from build123d import *

# Parameters (mm, degrees)
BOSS_EXTRUDE1_DEPTH = 2


with BuildPart() as part:
    # Sketch1 → Boss-Extrude1 (new body)
    with BuildSketch(Plane.XY):
        with BuildLine():
            Line((5, 6.009754879), (-15, 6.009754879))
            ThreePointArc((-15, 6.009754879), (-21.009754879, 0), (-15, -6.009754879))
            Line((-15, -6.009754879), (5, -6.009754879))
            Line((5, -6.009754879), (5, 6.009754879))
        make_face()
        with BuildLine():
            ThreePointArc((-12.450490243, -2.75), (-18.75, 0), (-12.450490243, 2.75))
            Line((-12.450490243, 2.75), (0, 2.25))
            ThreePointArc((0, 2.25), (1.590990258, 1.590990258), (2.25, 0))
            ThreePointArc((2.25, 0), (1.590990258, -1.590990258), (0, -2.25))
            Line((0, -2.25), (-12.450490243, -2.75))
        make_face(mode=Mode.SUBTRACT)
    extrude(amount=BOSS_EXTRUDE1_DEPTH)


solid = part.part
Check sheet for the modelled part. Datum: model origin and axes. Units: mm. A direction names the side the tool comes from. Coordinates: 2 decimals unless noted, no trailing zeros. Loops run counter-clockwise (first coordinate to the right, second up) from the corner with the lowest first, then second, coordinate; pieces in that order, holes last. Notation, with made-up numbers: (1, 86.25) -> (42, 86.25) arc R18 cw to (42, 117.25) -> close; hole circle Ø4 at (-10.5, 5). An arc over 180 degrees is marked (long way). Answer in a Markdown table with one row per item.
1. Release check for a two-part mould opening along X. For faces 3 (the face through (-6.312, 2.504, 0.986)), 4 (the face through (-5, 6.01, 1)), 5 (the face through (-21.01, 0.13, 0.99)) record: released by +X, released by -X, zero draft, split by the parting line, or undercut.
Check values:
| item | result |
|---|---|
| face 3 | undercut |
| face 4 | zero draft |
| face 5 | released by -X |
2. Go/stop test with a flat-tipped pin: pin 1 (1 mm diameter, centred on x = 1.5, y = -0.5, fed in from -Z) (3 decimals). Record where the tip stops, or that it passes through.
Check values:
| item | result |
|---|---|
| pin 1 | passes through |
3. Access from +Z, -Z, +X, -X, +Y, -Y to the whole of each face (thin tool, end or side, straight path). Record for faces 1 (the face through (-6.138, -2.496, 0.986)), 2 (the face through (-5, -6.01, 1)).
Check values:
| item | result |
|---|---|
| face 1 | +Z, -Z |
| face 2 | +Z, -Z, +X, -X, -Y |
4. Sectioned sample at A-A, the plane z = 0.3. Record the boundary of the cut face in (x, y).
Check values:
| item | result |
|---|---|
| outline | (-15, -6.01) -> (5, -6.01) -> (5, 6.01) -> (-15, 6.01) arc R6.01 ccw to start; hole (-12.45, -2.75) -> (0, -2.25) arc R2.25 ccw to (0, 2.25) -> (-12.45, 2.75) arc R3.75 ccw (long way) to start |
5. Sectioned sample at D-D, the plane y = -4. Record the boundary of the cut face in (x, z), then the cut area to 3 significant figures.
Check values:
| item | result |
|---|---|
| outline | (-19.49, 0) -> (5, 0) -> (5, 2) -> (-19.49, 2) -> close |
| area | 49.0 mm2 |
6. Material ranges on line 1 along Y through (x, z) = (-15, 1.4); line 2 along X through (y, z) = (1.5, 0.65); line 3 along Y through (x, z) = (-1.25, 0.3), recorded low to high. Write a range as [from, to].
Check values:
| item | result |
|---|---|
| line 1 | y = [-6.01, -3.75], [3.75, 6.01] |
| line 2 | x = [-20.82, -18.44], [1.68, 5] |
| line 3 | y = [-6.01, -2.3], [2.3, 6.01] |
7. Sectioned sample at B-B, the plane x = -5. Record the boundary of the cut face in (y, z), then the cut area to 3 significant figures.
Check values:
| item | result |
|---|---|
| outline | (-6.01, 0) -> (-2.45, 0) -> (-2.45, 2) -> (-6.01, 2) -> close; (2.45, 0) -> (6.01, 0) -> (6.01, 2) -> (2.45, 2) -> close |
| area | 14.2 mm2 |
8. Sectioned sample at C-C, the plane y = 3.5. Record the boundary of the cut face in (x, z).
Check values:
| item | result |
|---|---|
| outline | (-19.89, 0) -> (-16.35, 0) -> (-16.35, 2) -> (-19.89, 2) -> close; (-13.65, 0) -> (5, 0) -> (5, 2) -> (-13.65, 2) -> close |
